Read the model definition and answer for the solid it produces. Units are mm, in the model's axes. A direction names the side the tool comes from. Give positions to 0.01 mm unless a question says otherwise; leave off trailing zeros. Order: outer loops, then holes, each group sorted by start corner. A loop starts at its lowest first (then second) coordinate and runs counter-clockwise, first axis right, second up.
Item 1: Which of the six approach directions +Z, -Z, +X, -X, +Y, -Y give full straight-line access (tool end or side, diameter ignored) to faces 1 (the face through (6.5, 10, -8)), 2 (the face through (-3.1, 0, -8))?
Item 2: Given pin 1 Ø5.5 at (y, z) = (0, 14) entering from +X; pin 2 Ø12 at (x, y) = (11.5, 20.5) entering from +Z; pin 3 Ø8 at (y, z) = (14, 8) entering from +X; pin 4 Ø2 at (x, y) = (13.5, 4.5) entering from -Z, each flat-ended and moving along its own axis, determine where each tip first touches the part or whether it passes through.
Item 3: Find the intervals of material crossed by line 1 along Y through (x, z) = (-0.8, 0); line 2 along Y through (x, z) = (19.25, 0); line 3 along Z through (x, y) = (7.5, 13.5), in increasing order.
Item 4: The mould has two halves that part along Z. Classify faces 3 (the face through (23, 8, 0)), 4 (the face through (6.5, 1, 16)): +Z half, -Z half, draft (parallel to the pull), parting line (faces both ways), or undercut.
Item 5: A cutting plane is placed at A-A (y = 0). State how many separate pieces and enclosed holes the cut face has, plus the area to 3 significant figures.
Item 6: A cutting plane is placed at D-D (z = 14). Write down the section's boundary in (x, y) (3 decimals).
Item 7: A cutting plane is placed at B-B (y = 22.25). Write down the section's boundary in (x, z), plus the area to 3 significant figures.
from build123d import *

# Parameters (mm, degrees)
SKETCH13_R          = 35
SKETCH13_R_2        = 7.5
BOSS_EXTRUDE1_DEPTH = 23
SKETCH14_R          = 2.05
CUT_EXTRUDE1_DEPTH  = 55.580216196
SKETCH16_R          = 2.85
SKETCH16_R_2        = 2.05
CUT_EXTRUDE2_DEPTH  = 16.5
SKETCH16_4_R        = 2.85
SKETCH16_4_R_2      = 2.05
CUT_EXTRUDE3_DEPTH  = 8.5
SKETCH18_R          = 35
SKETCH18_R_2        = 7.5
SKETCH18_R_3        = 2.05
BOSS_EXTRUDE2_DEPTH = 3.1
SKETCH19_R          = 3.625
CUT_EXTRUDE4_DEPTH  = 9.5


with BuildPart() as part:
    # Sketch13 → Boss-Extrude1 (new body)
    with BuildSketch(Plane(origin=(0, 0, 0), x_dir=(0, 0, -1), z_dir=(1, 0, 0))):
        Circle(SKETCH13_R)
        Circle(SKETCH13_R_2, mode=Mode.SUBTRACT)
    extrude(amount=BOSS_EXTRUDE1_DEPTH)

    # Sketch14 → Cut-Extrude1 (cut, through all)
    with BuildSketch(Plane(origin=(23, 0, 0), x_dir=(0, 0, -1), z_dir=(1, 0, 0))):
        with Locations((14, 0)):
            Circle(SKETCH14_R)
        with Locations((19.269065234, -11.125)):
            Circle(SKETCH14_R)
        with Locations((7, 12.124355653)):
            Circle(SKETCH14_R)
        with Locations((19.269065234, 11.125)):
            Circle(SKETCH14_R)
        with Locations((-7, 12.124355653)):
            Circle(SKETCH14_R)
        with Locations((0, 22.25)):
            Circle(SKETCH14_R)
        with Locations((-14, 0)):
            Circle(SKETCH14_R)
        with Locations((-19.269065234, 11.125)):
            Circle(SKETCH14_R)
        with Locations((-7, -12.124355653)):
            Circle(SKETCH14_R)
        with Locations((-19.269065234, -11.125)):
            Circle(SKETCH14_R)
        with Locations((7, -12.124355653)):
            Circle(SKETCH14_R)
        with Locations((0, -22.25)):
            Circle(SKETCH14_R)
    extrude(amount=-CUT_EXTRUDE1_DEPTH, mode=Mode.SUBTRACT)

    # Sketch16 → Cut-Extrude2 (cut)
    # profile 1 of 11: a face of its own
    with BuildSketch(Plane(origin=(23, 0, 0), x_dir=(0, 0, -1), z_dir=(1, 0, 0))):
        with Locations((-14, 0)):
            Circle(SKETCH16_R)
        with Locations((-14, 0)):
            Circle(SKETCH16_R_2, mode=Mode.SUBTRACT)
    # profile 2 of 11: a face of its own
    with BuildSketch(Plane(origin=(23, 0, 0), x_dir=(0, 0, -1), z_dir=(1, 0, 0))):
        with Locations((-14, 0)):
            Circle(SKETCH16_R_2)
    # profile 3 of 11: a face of its own
    with BuildSketch(Plane(origin=(23, 0, 0), x_dir=(0, 0, -1), z_dir=(1, 0, 0))):
        with Locations((-7, -12.124355653)):
            Circle(SKETCH16_R)
        with Locations((-7, -12.124355653)):
            Circle(SKETCH16_R_2, mode=Mode.SUBTRACT)
    # profile 4 of 11: a face of its own
    with BuildSketch(Plane(origin=(23, 0, 0), x_dir=(0, 0, -1), z_dir=(1, 0, 0))):
        with Locations((-7, -12.124355653)):
            Circle(SKETCH16_R_2)
    # profile 5 of 11: a face of its own
    with BuildSketch(Plane(origin=(23, 0, 0), x_dir=(0, 0, -1), z_dir=(1, 0, 0))):
        with Locations((7, -12.124355653)):
            Circle(SKETCH16_R)
        with Locations((7, -12.124355653)):
            Circle(SKETCH16_R_2, mode=Mode.SUBTRACT)
    # profile 6 of 11: a face of its own
    with BuildSketch(Plane(origin=(23, 0, 0), x_dir=(0, 0, -1), z_dir=(1, 0, 0))):
        with Locations((7, -12.124355653)):
            Circle(SKETCH16_R_2)
    # profile 7 of 11: a face of its own
    with BuildSketch(Plane(origin=(23, 0, 0), x_dir=(0, 0, -1), z_dir=(1, 0, 0))):
        with Locations((14, 0)):
            Circle(SKETCH16_R_2)
    # profile 8 of 11: a face of its own
    with BuildSketch(Plane(origin=(23, 0, 0), x_dir=(0, 0, -1), z_dir=(1, 0, 0))):
        with Locations((7, 12.124355653)):
            Circle(SKETCH16_R)
        with Locations((7, 12.124355653)):
            Circle(SKETCH16_R_2, mode=Mode.SUBTRACT)
    # profile 9 of 11: a face of its own
    with BuildSketch(Plane(origin=(23, 0, 0), x_dir=(0, 0, -1), z_dir=(1, 0, 0))):
        with Locations((7, 12.124355653)):
            Circle(SKETCH16_R_2)
    # profile 10 of 11: a face of its own
    with BuildSketch(Plane(origin=(23, 0, 0), x_dir=(0, 0, -1), z_dir=(1, 0, 0))):
        with Locations((-7, 12.124355653)):
            Circle(SKETCH16_R)
    # profile 11 of 11: a face of its own
    with BuildSketch(Plane(origin=(23, 0, 0), x_dir=(0, 0, -1), z_dir=(1, 0, 0))):
        with Locations((14, 0)):
            Circle(SKETCH16_R)
    extrude(amount=-CUT_EXTRUDE2_DEPTH, mode=Mode.SUBTRACT)

    # Sketch16_4 → Cut-Extrude3 (cut)
    # profile 1 of 12: a face of its own
    with BuildSketch(Plane(origin=(23, 0, 0), x_dir=(0, 0, -1), z_dir=(1, 0, 0))):
        with Locations((-19.269065234, -11.125)):
            Circle(SKETCH16_4_R)
        with Locations((-19.269065234, -11.125)):
            Circle(SKETCH16_4_R_2, mode=Mode.SUBTRACT)
    # profile 2 of 12: a face of its own
    with BuildSketch(Plane(origin=(23, 0, 0), x_dir=(0, 0, -1), z_dir=(1, 0, 0))):
        with Locations((-19.269065234, 11.125)):
            Circle(SKETCH16_4_R)
        with Locations((-19.269065234, 11.125)):
            Circle(SKETCH16_4_R_2, mode=Mode.SUBTRACT)
    # profile 3 of 12: a face of its own
    with BuildSketch(Plane(origin=(23, 0, 0), x_dir=(0, 0, -1), z_dir=(1, 0, 0))):
        with Locations((-19.269065234, 11.125)):
            Circle(SKETCH16_4_R_2)
    # profile 4 of 12: a face of its own
    with BuildSketch(Plane(origin=(23, 0, 0), x_dir=(0, 0, -1), z_dir=(1, 0, 0))):
        with Locations((-19.269065234, -11.125)):
            Circle(SKETCH16_4_R_2)
    # profile 5 of 12: a face of its own
    with BuildSketch(Plane(origin=(23, 0, 0), x_dir=(0, 0, -1), z_dir=(1, 0, 0))):
        with Locations((0, 22.25)):
            Circle(SKETCH16_4_R)
        with Locations((0, 22.25)):
            Circle(SKETCH16_4_R_2, mode=Mode.SUBTRACT)
    # profile 6 of 12: a face of its own
    with BuildSketch(Plane(origin=(23, 0, 0), x_dir=(0, 0, -1), z_dir=(1, 0, 0))):
        with Locations((0, 22.25)):
            Circle(SKETCH16_4_R_2)
    # profile 7 of 12: a face of its own
    with BuildSketch(Plane(origin=(23, 0, 0), x_dir=(0, 0, -1), z_dir=(1, 0, 0))):
        with Locations((19.269065234, 11.125)):
            Circle(SKETCH16_4_R_2)
    # profile 8 of 12: a face of its own
    with BuildSketch(Plane(origin=(23, 0, 0), x_dir=(0, 0, -1), z_dir=(1, 0, 0))):
        with Locations((19.269065234, -11.125)):
            Circle(SKETCH16_4_R)
        with Locations((19.269065234, -11.125)):
            Circle(SKETCH16_4_R_2, mode=Mode.SUBTRACT)
    # profile 9 of 12: a face of its own
    with BuildSketch(Plane(origin=(23, 0, 0), x_dir=(0, 0, -1), z_dir=(1, 0, 0))):
        with Locations((19.269065234, -11.125)):
            Circle(SKETCH16_4_R_2)
    # profile 10 of 12: a face of its own
    with BuildSketch(Plane(origin=(23, 0, 0), x_dir=(0, 0, -1), z_dir=(1, 0, 0))):
        with Locations((0, -22.25)):
            Circle(SKETCH16_4_R_2)
    # profile 11 of 12: a face of its own
    with BuildSketch(Plane(origin=(23, 0, 0), x_dir=(0, 0, -1), z_dir=(1, 0, 0))):
        with Locations((19.269065234, 11.125)):
            Circle(SKETCH16_4_R)
    # profile 12 of 12: a face of its own
    with BuildSketch(Plane(origin=(23, 0, 0), x_dir=(0, 0, -1), z_dir=(1, 0, 0))):
        with Locations((0, -22.25)):
            Circle(SKETCH16_4_R)
    extrude(amount=-CUT_EXTRUDE3_DEPTH, mode=Mode.SUBTRACT)

    # Sketch18 → Boss-Extrude2 (add)
    with BuildSketch(Plane.ZY):
        Circle(SKETCH18_R)
        Circle(SKETCH18_R_2, mode=Mode.SUBTRACT)
        with Locations(Location((-14, 0, 0), (0, 0, 180))):
            Circle(SKETCH18_R_3, mode=Mode.SUBTRACT)
        with Locations(Location((-19.269065234, 11.125, 0), (0, 0, 180))):
            Circle(SKETCH18_R_3, mode=Mode.SUBTRACT)
        with Locations(Location((-7, 12.124355653, 0), (0, 0, 180))):
            Circle(SKETCH18_R_3, mode=Mode.SUBTRACT)
        with Locations(Location((0, 22.25, 0), (0, 0, 180))):
            Circle(SKETCH18_R_3, mode=Mode.SUBTRACT)
        with Locations(Location((7, 12.124355653, 0), (0, 0, 180))):
            Circle(SKETCH18_R_3, mode=Mode.SUBTRACT)
        with Locations(Location((19.269065234, 11.125, 0), (0, 0, 180))):
            Circle(SKETCH18_R_3, mode=Mode.SUBTRACT)
        with Locations(Location((14, 0, 0), (0, 0, 180))):
            Circle(SKETCH18_R_3, mode=Mode.SUBTRACT)
        with Locations(Location((19.269065234, -11.125, 0), (0, 0, 180))):
            Circle(SKETCH18_R_3, mode=Mode.SUBTRACT)
        with Locations(Location((7, -12.124355653, 0), (0, 0, 180))):
            Circle(SKETCH18_R_3, mode=Mode.SUBTRACT)
        with Locations(Location((0, -22.25, 0), (0, 0, 180))):
            Circle(SKETCH18_R_3, mode=Mode.SUBTRACT)
        with Locations(Location((-7, -12.124355653, 0), (0, 0, 180))):
            Circle(SKETCH18_R_3, mode=Mode.SUBTRACT)
        with Locations(Location((-19.269065234, -11.125, 0), (0, 0, 180))):
            Circle(SKETCH18_R_3, mode=Mode.SUBTRACT)
    extrude(amount=BOSS_EXTRUDE2_DEPTH)

    # Sketch19 → Cut-Extrude4 (cut)
    with BuildSketch(Plane(origin=(23, 0, 0), x_dir=(0, 0, -1), z_dir=(1, 0, 0))):
        with Locations((-7, 12.124355653)):
            Circle(SKETCH19_R)
        with Locations((7, 12.124355653)):
            Circle(SKETCH19_R)
        with Locations((14, 0)):
            Circle(SKETCH19_R)
        with Locations((7, -12.124355653)):
            Circle(SKETCH19_R)
        with Locations((-7, -12.124355653)):
            Circle(SKETCH19_R)
        with Locations((-14, 0)):
            Circle(SKETCH19_R)
    extrude(amount=-CUT_EXTRUDE4_DEPTH, mode=Mode.SUBTRACT)


solid = part.part
Response values:
1. face 1: +X
1. face 2: +Z, -Z, -X, +Y, -Y
2. pin 1: stops at x = 6.5
2. pin 2: stops at z = 31.86
2. pin 3: stops at x = 23
2. pin 4: stops at z = -34.82
3. line 1: y = -35 to -24.3, -20.2 to -7.5, 7.5 to 20.2, 24.3 to 35
3. line 2: y = -35 to -25.1, -19.4 to -7.5, 7.5 to 19.4, 25.1 to 35
3. line 3: z = -32.29 to -9.5, -4.5 to 4.5, 9.5 to 32.29
4. face 3: draft
4. face 4: undercut
5. separate pieces: 4
5. enclosed holes: 0
5. area: 1,140 mm2
6. outline: (-3.1, -32.078) - (23, -32.078) - (23, -3.625) - (13.5, -3.625) - (13.5, -2.85) - (6.5, -2.85) - (6.5, -2.05) - (-3.1, -2.05) - close; (-3.1, 2.05) - (6.5, 2.05) - (6.5, 2.85) - (13.5, 2.85) - (13.5, 3.625) - (23, 3.625) - (23, 32.078) - (-3.1, 32.078) - close
7. outline: (-3.1, -27.02) - (23, -27.02) - (23, -2.85) - (14.5, -2.85) - (14.5, -2.05) - (-3.1, -2.05) - close; (-3.1, 2.05) - (14.5, 2.05) - (14.5, 2.85) - (23, 2.85) - (23, 27.02) - (-3.1, 27.02) - close
7. area: 1,290 mm2
